```python
from build123d import *

# Parameters (mm, degrees)
SKETCH1_W           = 90
SKETCH1_H           = 25
SKETCH1_R           = 4
SKETCH1_R_2         = 1.5
BOSS_EXTRUDE1_DEPTH = 2
SKETCH2_W           = 90
SKETCH2_H           = 42
SKETCH2_R           = 4
SKETCH2_R_2         = 1.5
BOSS_EXTRUDE2_DEPTH = 2


with BuildPart() as part:
    # Sketch1 → Boss-Extrude1 (new body)
    with BuildSketch(Plane(origin=(0, 0, 0), x_dir=(1, 0, 0), z_dir=(0, 1, 0))):
        Rectangle(SKETCH1_W, SKETCH1_H)
        Circle(SKETCH1_R, mode=Mode.SUBTRACT)
        with Locations((34.75, 0)):
            Circle(SKETCH1_R, mode=Mode.SUBTRACT)
        with Locations((0, 7)):
            Circle(SKETCH1_R_2, mode=Mode.SUBTRACT)
        with Locations((7, 0)):
            Circle(SKETCH1_R_2, mode=Mode.SUBTRACT)
        with Locations((-7, 0)):
            Circle(SKETCH1_R_2, mode=Mode.SUBTRACT)
        with Locations((0, -7)):
            Circle(SKETCH1_R_2, mode=Mode.SUBTRACT)
        with Locations((-34.75, 0)):
            Circle(SKETCH1_R, mode=Mode.SUBTRACT)
        with Locations((34.75, 7)):
            Circle(SKETCH1_R_2, mode=Mode.SUBTRACT)
        with Locations((41.75, 0)):
            Circle(SKETCH1_R_2, mode=Mode.SUBTRACT)
        with Locations((34.75, -7)):
            Circle(SKETCH1_R_2, mode=Mode.SUBTRACT)
        with Locations((27.75, 0)):
            Circle(SKETCH1_R_2, mode=Mode.SUBTRACT)
        with Locations((-34.75, 7)):
            Circle(SKETCH1_R_2, mode=Mode.SUBTRACT)
        with Locations((-27.75, 0)):
            Circle(SKETCH1_R_2, mode=Mode.SUBTRACT)
        with Locations((-34.75, -7)):
            Circle(SKETCH1_R_2, mode=Mode.SUBTRACT)
        with Locations((-41.75, 0)):
            Circle(SKETCH1_R_2, mode=Mode.SUBTRACT)
    extrude(amount=BOSS_EXTRUDE1_DEPTH)

    # Sketch2 → Boss-Extrude2 (add)
    with BuildSketch(Plane.XY.offset(12.5)):
        with Locations((0, 21)):
            Rectangle(SKETCH2_W, SKETCH2_H)
        with Locations((0, 30.08)):
            Circle(SKETCH2_R, mode=Mode.SUBTRACT)
        with Locations((0, 37.08)):
            Circle(SKETCH2_R_2, mode=Mode.SUBTRACT)
        with Locations((7, 30.08)):
            Circle(SKETCH2_R_2, mode=Mode.SUBTRACT)
        with Locations((0, 23.08)):
            Circle(SKETCH2_R_2, mode=Mode.SUBTRACT)
        with Locations((-7, 30.08)):
            Circle(SKETCH2_R_2, mode=Mode.SUBTRACT)
        with Locations((34.75, 30.08)):
            Circle(SKETCH2_R, mode=Mode.SUBTRACT)
        with Locations((34.75, 37.08)):
            Circle(SKETCH2_R_2, mode=Mode.SUBTRACT)
        with Locations((41.75, 30.08)):
            Circle(SKETCH2_R_2, mode=Mode.SUBTRACT)
        with Locations((34.75, 23.08)):
            Circle(SKETCH2_R_2, mode=Mode.SUBTRACT)
        with Locations((27.75, 30.08)):
            Circle(SKETCH2_R_2, mode=Mode.SUBTRACT)
        with Locations((-34.75, 30.08)):
            Circle(SKETCH2_R, mode=Mode.SUBTRACT)
        with Locations((-34.75, 37.08)):
            Circle(SKETCH2_R_2, mode=Mode.SUBTRACT)
        with Locations((-27.75, 30.08)):
            Circle(SKETCH2_R_2, mode=Mode.SUBTRACT)
        with Locations((-34.75, 23.08)):
            Circle(SKETCH2_R_2, mode=Mode.SUBTRACT)
        with Locations((-41.75, 30.08)):
            Circle(SKETCH2_R_2, mode=Mode.SUBTRACT)
        with Locations((13.75, 37.08)):
            Circle(SKETCH2_R_2, mode=Mode.SUBTRACT)
        with Locations((-13.75, 37.08)):
            Circle(SKETCH2_R_2, mode=Mode.SUBTRACT)
    extrude(amount=BOSS_EXTRUDE2_DEPTH)

    # Mirror1: part across plane


with BuildPart() as part_1:
    add(part.part)
    add(part.part.mirror(Plane.XY))


solid = part_1.part
```
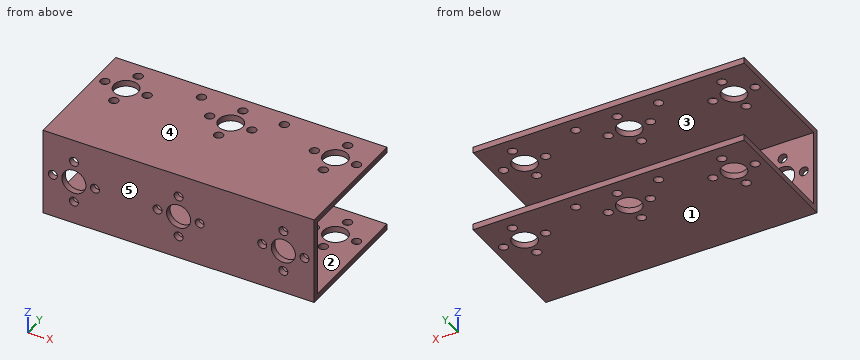
The listing builds one solid part. Answer for the finished solid, in the listing's coordinates (mm). Face numbers are marked on the shaded views. A direction names the side the tool comes from. Coordinates: 2 decimals unless noted, no trailing zeros. Write each loop counter-clockwise with the first axis right and the second up, starting at its lowest first coordinate (ties: lowest second). Pieces come first, ordered by that corner, then holes. Notation, with made-up numbers: M 88,74.25 L 129,74.25 A27 ccw 129,101.25 Z; hole C -11,23 d4. An arc over 180 degrees is marked long. Use a Markdown table: item, result. Add a question column.
1. Given P1, Ø8, axis at x = 18.5, z = 1.5, coming from the +Y side; P2, Ø2.5, axis at x = 0, z = 7, coming from the -Y side (1 decimal), each flat-ended and moving along its own axis, determine where each tip first touches the part or whether it passes through.
2. Section B-B (x = -27.75) is taken. Give the vertices of the cut face in (y, z).
3. Which of the six approach directions +Z, -Z, +X, -X, +Y, -Y give full straight-line access (tool end or side, diameter ignored) to the marked faces 1 and 2?
4. Straight lines are drawn through the part: line 1 along Y through (x, z) = (34.75, -13.3); line 2 along Z through (x, y) = (-34.75, 1.4); line 3 along Z through (x, y) = (-29, 38). For each, find the intervals that lie inside material, in ascending order. Write a range as [from, to].
5. Section A-A (y = 18) is taken. Give the vertices of the cut face in (x, z).
6. For a pull along Z with two mould halves and no side action, classify the marked faces 3, 4 and 5 as +Z half, -Z half, draft (parallel to the pull), parting line (faces both ways), or undercut.
7. Section D-D (y = 23.08) is taken. Count the separate pieces of the cut face and the enclosed holes in it, plus the area to 3 significant figures.
8. Section C-C (z = -7) is taken. Give the vertices of the cut face in (x, y), plus the area to 3 significant figures.
Data:
| question | item | result |
|---|---|---|
| 1 | P1 | stops at y = 2 |
| 1 | P2 | passes through |
| 2 | outline | M 0,-14.5 L 28.58,-14.5 L 28.58,-12.5 L 2,-12.5 L 2,-1.5 L 0,-1.5 Z; M 0,1.5 L 2,1.5 L 2,12.5 L 28.58,12.5 L 28.58,14.5 L 0,14.5 Z; M 31.58,-14.5 L 42,-14.5 L 42,-12.5 L 31.58,-12.5 Z; M 31.58,12.5 L 42,12.5 L 42,14.5 L 31.58,14.5 Z |
| 3 | face 1 | -Z, +X, -X, +Y, -Y |
| 3 | face 2 | +X, -X, +Y |
| 4 | line 1 | y = [0, 21.58], [24.58, 26.08], [34.08, 35.58], [38.58, 42] |
| 4 | line 2 | z = [-14.5, -8.5], [-5.5, -4], [4, 5.5], [8.5, 14.5] |
| 4 | line 3 | z = [-14.5, -12.5], [12.5, 14.5] |
| 5 | outline | M -45,-14.5 L 45,-14.5 L 45,-12.5 L -45,-12.5 Z; M -45,12.5 L 45,12.5 L 45,14.5 L -45,14.5 Z |
| 6 | face 3 | undercut |
| 6 | face 4 | +Z half |
| 6 | face 5 | draft |
| 7 | separate pieces | 8 |
| 7 | enclosed holes | 0 |
| 7 | area | 324 mm2 |
| 8 | outline | M -45,0 L -36.25,0 L -36.25,2 L -45,2 Z; M -33.25,0 L -1.5,0 L -1.5,2 L -33.25,2 Z; M 1.5,0 L 33.25,0 L 33.25,2 L 1.5,2 Z; M 36.25,0 L 45,0 L 45,2 L 36.25,2 Z |
| 8 | area | 162 mm2 |
